```python
from build123d import *

# Parameters (mm, degrees)
PLATEOUTLINE_W      = 80
PLATEOUTLINE_H      = 80
BOSS_EXTRUDE1_DEPTH = 6.2738
RAILGUIDES_R        = 4.7625
CUT_EXTRUDE1_DEPTH  = 10
CUT_EXTRUDE2_START  = 5
FUELGRAINMOUNTING_R = 30.1625
CUT_EXTRUDE2_DEPTH  = 5
GASINTAKE_R         = 27.051
CUT_EXTRUDE3_DEPTH  = 5
CUT_EXTRUDE4_START  = 5
SKETCH1_R           = 30.1625
SKETCH1_R_2         = 28.575
CUT_EXTRUDE4_DEPTH  = 1.143


with BuildPart() as part:
    # plateOutline → Boss-Extrude1 (new body)
    with BuildSketch(Plane(origin=(0, 0, 0), x_dir=(1, 0, 0), z_dir=(0, 1, 0))):
        Rectangle(PLATEOUTLINE_W, PLATEOUTLINE_H)
    extrude(amount=BOSS_EXTRUDE1_DEPTH)

    # railGuides → Cut-Extrude1 (cut)
    with BuildSketch(Plane(origin=(0, 0, 0), x_dir=(1, 0, 0), z_dir=(0, 1, 0))):
        with Locations((-32.5, 32.5)):
            Circle(RAILGUIDES_R)
        with Locations((32.5, 32.5)):
            Circle(RAILGUIDES_R)
        with Locations((32.5, -32.5)):
            Circle(RAILGUIDES_R)
        with Locations((-32.5, -32.5)):
            Circle(RAILGUIDES_R)
    extrude(amount=CUT_EXTRUDE1_DEPTH, mode=Mode.SUBTRACT)

    # FuelGrainMounting → Cut-Extrude2 (cut)
    with BuildSketch(Plane(origin=(0, 0, 0), x_dir=(1, 0, 0), z_dir=(0, 1, 0)).offset(CUT_EXTRUDE2_START)):
        Circle(FUELGRAINMOUNTING_R)
    extrude(amount=CUT_EXTRUDE2_DEPTH, mode=Mode.SUBTRACT)

    # GasIntake → Cut-Extrude3 (cut)
    with BuildSketch(Plane(origin=(0, 0, 0), x_dir=(1, 0, 0), z_dir=(0, 1, 0))):
        Circle(GASINTAKE_R)
    extrude(amount=CUT_EXTRUDE3_DEPTH, mode=Mode.SUBTRACT)

    # Sketch1 → Cut-Extrude4 (cut)
    with BuildSketch(Plane(origin=(0, 0, 0), x_dir=(1, 0, 0), z_dir=(0, 1, 0)).offset(CUT_EXTRUDE4_START)):
        Circle(SKETCH1_R)
        Circle(SKETCH1_R_2, mode=Mode.SUBTRACT)
    extrude(amount=-CUT_EXTRUDE4_DEPTH, mode=Mode.SUBTRACT)


solid = part.part
```
Source: CAD feature listing. Evaluate the final solid. Frame: model axes, mm. A direction names the side the tool comes from. Coordinates: 2 decimals unless noted, no trailing zeros. Loops run counter-clockwise (first coordinate to the right, second up) from the corner with the lowest first, then second, coordinate; pieces in that order, holes last. Notation, with made-up numbers: M 16.5,23.25 L 50.5,23.25 A19 cw 50.5,28.25 Z; hole C 15.25,44.5 d7. An arc over 180 degrees is marked long. Put each result on its own line as item: value. Start each with the question number.
1) Pull-direction query (X, two-part tool) for faces 1 (the face through (-1, 3, -40)), 2 (the face through (-30.133, 5.048, -1.326)), 3 (the face through (40, 3, 1)); classes: pulls with the +X half, pulls with the -X half, needs draft (parallel to the pull), parting line crosses it, or undercut.
2) Cut plane D-D on x = 0. Return the cut outline in (y, z) (1 decimal), then the cut area to 3 significant figures.
3) Contact query for flat-ended pins moving along their axis: pin 1 Ø18 at (x, z) = (-1, 13) entering from +Y; pin 2 Ø10 at (x, z) = (-13.5, -18) entering from +Y. Output: stop coordinate, or through.
4) Cut plane A-A on x = 32.5. Return the cut outline in (y, z).
5) Cut plane B-B on y = 1.75. Return the cut outline in (x, z) (1 decimal).
6) Ray query, L1, parallel to X at y = 2, z = 32.5; L2, parallel to Z at x = 0, y = 5.2. Return the intervals inside material, ascending. Write a range as from..to.
7) Reachability of faces 4 (the face through (-28.547, 4.437, -1.256)), 5 (the face through (37.043, 3.093, -33.931)) from +Z, -Z, +X, -X, +Y, -Y: full face, straight path, thin tool, end or side. Return the list, or none.
8) Cut plane C-C on z = 32.5. Return the cut outline in (x, y).
The answers:
1. face 1: needs draft
1. face 2: undercut
1. face 3: pulls with the +X half
2. outline: M 0,-40 L 6.3,-40 L 6.3,-30.2 L 3.9,-30.2 L 3.9,-28.6 L 5,-28.6 L 5,-27.1 L 0,-27.1 Z; M 0,27.1 L 5,27.1 L 5,28.6 L 3.9,28.6 L 3.9,30.2 L 6.3,30.2 L 6.3,40 L 0,40 Z
2. area: 151 mm²
3. pin 1: passes through
3. pin 2: stops at y = 5
4. outline: M 0,-40 L 6.27,-40 L 6.27,-37.26 L 0,-37.26 Z; M 0,-27.74 L 6.27,-27.74 L 6.27,27.74 L 0,27.74 Z; M 0,37.26 L 6.27,37.26 L 6.27,40 L 0,40 Z
5. outline: M -40,-40 L 40,-40 L 40,40 L -40,40 Z; hole C -32.5,-32.5 d9.5; hole C -32.5,32.5 d9.5; hole C 0,0 d54.1; hole C 32.5,-32.5 d9.5; hole C 32.5,32.5 d9.5
6. L1: x = -40..-37.26, -27.74..27.74, 37.26..40
6. L2: z = -40..-30.16, 30.16..40
7. face 4: +Y
7. face 5: +Y, -Y
8. outline: M -40,0 L -37.26,0 L -37.26,6.27 L -40,6.27 Z; M -27.74,0 L 27.74,0 L 27.74,6.27 L -27.74,6.27 Z; M 37.26,0 L 40,0 L 40,6.27 L 37.26,6.27 Z
